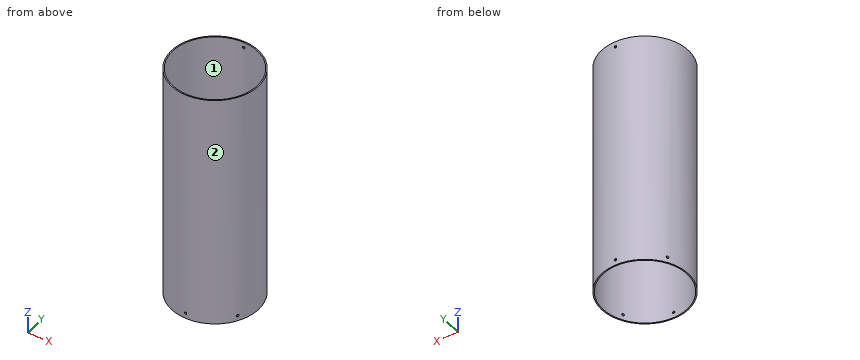
from build123d import *

# Parameters (mm, degrees)
SKETCH1_R           = 78.359
SKETCH1_R_2         = 76.2
BOSS_EXTRUDE1_DEPTH = 426.75
SKETCH5_W           = 2.25
SKETCH5_H           = 78.359
CIRPATTERN1_COUNT   = 6
SKETCH7_W           = 2.25
SKETCH7_H           = 78.359


with BuildPart() as part:
    # Sketch1 → Boss-Extrude1 (new body)
    with BuildSketch(Plane.XY):
        Circle(SKETCH1_R)
        Circle(SKETCH1_R_2, mode=Mode.SUBTRACT)
    extrude(amount=BOSS_EXTRUDE1_DEPTH)

    # Sketch5 → M4 Clearance Hole2 (revolve, cut)
    with BuildSketch(Plane(origin=(0, 0, 10), x_dir=(0, 0, 1), z_dir=(1, 0, 0))):
        with Locations((1.125, 39.1795)):
            Rectangle(SKETCH5_W, SKETCH5_H)
    m4_clearance_hole2 = revolve(axis=Axis((0, 6.35, 10), (0, -1, 0)), mode=Mode.SUBTRACT)

    # CirPattern1: M4 Clearance Hole2 ×6 about axis
    cirpattern1_axis = Axis((0, 0, 426.75), (0, 0, -1))
    for i in range(1, CIRPATTERN1_COUNT):
        add(m4_clearance_hole2.rotate(cirpattern1_axis, i * 360 / CIRPATTERN1_COUNT), mode=Mode.SUBTRACT)

    # Sketch7 → M4 Clearance Hole3 (revolve, cut)
    with BuildSketch(Plane(origin=(0, 0, 416.75), x_dir=(0, 0, -1), z_dir=(1, 0, 0))):
        with Locations((1.125, 39.1795)):
            Rectangle(SKETCH7_W, SKETCH7_H)
    revolve(axis=Axis((0, -6.35, 416.75), (0, 1, 0)), mode=Mode.SUBTRACT)


solid = part.part
Work out the finished part from the listing and answer in its coordinate system (mm). Face numbers are marked on the shaded views. Round coordinates to 2 decimals unless told otherwise and drop trailing zeros. Order: outer loops, then holes, each group sorted by start corner. A loop starts at its lowest first (then second) coordinate and runs counter-clockwise, first axis right, second up. Notation, with made-up numbers: M 61.25,28 L 99.25,28 A22 cw 99.25,54 Z; hole C 20,0.5 d3. An arc over 180 degrees is marked long. Put each result on its own line as item: value. Start each with the question number.
Q1. Section A-A, the plane y = 0 is taken. Write down the section's boundary in (x, z).
Q2. Straight lines are drawn through the part: L1, parallel to Z at x = 0, y = 76.9; L2, parallel to Y at x = 0, z = 150.5; L3, parallel to X at y = -2.5, z = 53.5. For each, find the intervals that lie inside material, in ascending order. Write a range as [from, to].
Q3. Flat-ended cylindrical pins translate along their axes: pin 1 (6 mm diameter, centred on y = 56, z = 336.5, fed in from -X); pin 2 (5 mm diameter, centred on x = -27, z = 235.5, fed in from -Y); pin 3 (12 mm diameter, centred on y = 45, z = 381.5, fed in from -X). Find the tip coordinate at first contact, or state that the pin passes through.
Q4. For a pull along Y with two mould halves and no side action, classify the marked faces 1 and 2 as pulls with the +Y half, pulls with the -Y half, needs draft (parallel to the pull), parting line crosses it, or undercut.
Q5. Section B-B, the plane x = -38.5 is taken. Write down the section's boundary in (y, z).
Q6. Section C-C, the plane z = 231 is taken. Write down the section's boundary in (x, y).
Findings below:
1. outline: M -78.36,0 L -76.2,0 L -76.2,426.75 L -78.36,426.75 Z; M 76.2,0 L 78.36,0 L 78.36,426.75 L 76.2,426.75 Z
2. L1: z = [0, 7.75], [12.25, 414.5], [419, 426.75]
2. L2: y = [-78.36, -76.2], [76.2, 78.36]
2. L3: x = [-78.32, -76.16], [76.16, 78.32]
3. pin 1: stops at x = -57.72
3. pin 2: stops at y = -74.43
3. pin 3: stops at x = -67.96
4. face 1: undercut
4. face 2: parting line crosses it
5. outline: M -68.25,0 L -65.76,0 L -65.76,426.75 L -68.25,426.75 Z; M 65.76,0 L 68.25,0 L 68.25,426.75 L 65.76,426.75 Z
6. outline: C 0,0 d156.72; hole C 0,0 d152.4
